For this review, use the dimensioned drawing (mm, ordinates from the lowest corner) and the shaded views. Round coordinates to 2 decimals unless told otherwise and drop trailing zeros. Write each loop counter-clockwise with the first axis right and the second up, starting at its lowest first coordinate (ties: lowest second). Pieces come first, ordered by that corner, then holes. Notation, with made-up numbers: M -35.75,-4 L -16.75,-4 A21 ccw -16.75,6 Z; hole C -12.75,-12.5 d1. An arc over 180 degrees is marked long. Answer in a Markdown table with one row per item.
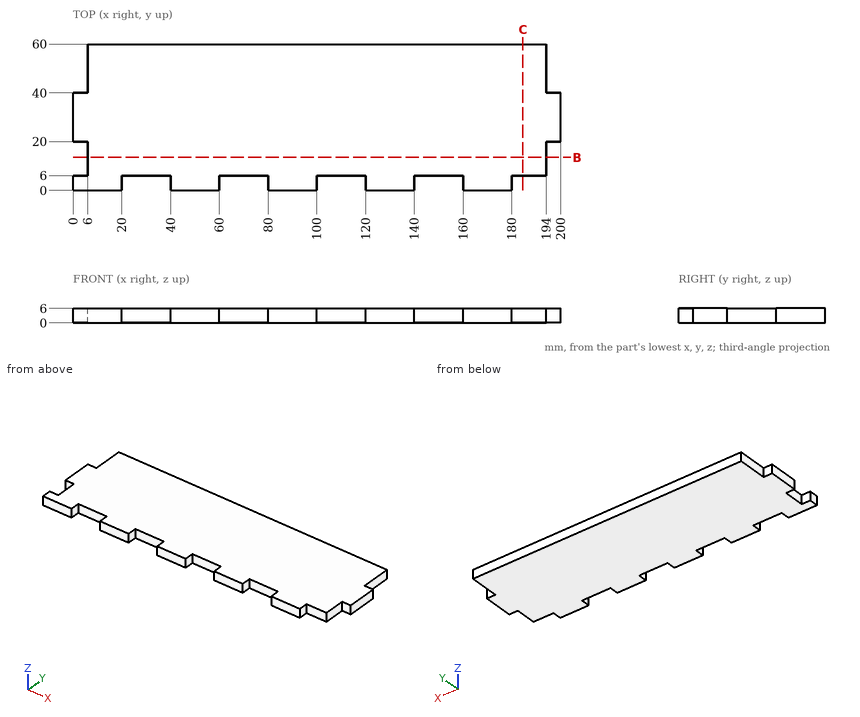
Q1. Insertion check: P1, Ø2, axis at y = 47.5, z = 5.5, coming from the -X side; P2, Ø1.8, axis at y = 54.5, z = 4.5, coming from the +X side; P3, Ø1, axis at x = 147, z = 2, coming from the -Y side. Each pin has a flat end and moves straight along its axis. Give the tip position at first contact, or say it passes through.
Found:
| item | result |
|---|---|
| P1 | x = 6 |
| P2 | x = 194 |
| P3 | y = 6 |
Q2. Take a section at C-C (x = 184.5). State the section outline as (y, z) points, then the cut area to 3 significant figures.
Found:
| item | result |
|---|---|
| outline | M 6,0 L 60,0 L 60,6 L 6,6 Z |
| area | 324 mm² |
Q3. For probe 1 along Y at (x, z) = (31.5, 2.15); probe 2 along X at (y, z) = (57, 3.5), list the stretches that pass through material, from the lowest coordinate up.
Found:
| item | result |
|---|---|
| probe 1 | 6 to 60 |
| probe 2 | 6 to 194 |
Q4. Take a section at B-B (y = 13.5). State the section outline as (x, z) points, then the cut area to 3 significant figures.
Found:
| item | result |
|---|---|
| outline | M 6,0 L 194,0 L 194,6 L 6,6 Z |
| area | 1,130 mm² |
